```python
from build123d import *

# Parameters (mm, degrees)
SKETCH1_W                       = 63.5
SKETCH1_H                       = 44.45
BOSS_EXTRUDE1_DEPTH             = 6.35
LPATTERN1_COUNT                 = 2
LPATTERN1_PITCH                 = 55.88
TAP_DRILL_FOR_6_32_TAP1_D       = 2.7051
TAP_DRILL_FOR_6_32_TAP1_DEPTH   = 6.35
TAP_DRILL_FOR_6_32_TAP1_TIP     = 0.81269403
TAP_DRILL_FOR_6_32_TAP2_D       = 2.7051
TAP_DRILL_FOR_6_32_TAP2_DEPTH   = 6.35
TAP_DRILL_FOR_6_32_TAP2_TIP     = 0.81269403
TAP_DRILL_FOR_1_2_13_TAP1_D     = 10.71626
TAP_DRILL_FOR_1_2_13_TAP1_DEPTH = 6.35
TAP_DRILL_FOR_1_2_13_TAP1_TIP   = 3.219489309


with BuildPart() as part:
    # Sketch1 → Boss-Extrude1 (new body)
    with BuildSketch(Plane(origin=(0, 0, 0), x_dir=(1, 0, 0), z_dir=(0, 1, 0))):
        with Locations((4.75259427, -18.964156798)):
            Rectangle(SKETCH1_W, SKETCH1_H)
    extrude(amount=BOSS_EXTRUDE1_DEPTH)

    # Sketch16 → Tap Drill for #4-40 Tap1 (revolve, cut)
    with BuildSketch(Plane(origin=(-23.18740573, 0, 18.964156798), x_dir=(0, 0, -1), z_dir=(1, 0, 0))):
        Polygon((0, 0), (0, 13.379152758), (1.1303, 12.7), (1.1303, 0), align=None)
    tap_drill_for_4_40_tap1 = revolve(axis=Axis((-23.18740573, -6.35, 18.964156798), (0, 1, 0)), mode=Mode.SUBTRACT)

    # LPattern1: Tap Drill for #4-40 Tap1 ×2
    with Locations(*[(i * LPATTERN1_PITCH, 0, 0) for i in range(1, LPATTERN1_COUNT)]):
        add(tap_drill_for_4_40_tap1, mode=Mode.SUBTRACT)

    # Tap Drill for #6-32 Tap1
    with Locations(Plane.XY.offset(41.189156798)):
        with Locations((23.80259427, 3.175), (-14.29740573, 3.175)):
            Hole(TAP_DRILL_FOR_6_32_TAP1_D / 2, depth=TAP_DRILL_FOR_6_32_TAP1_DEPTH)
            with Locations((0, 0, -(TAP_DRILL_FOR_6_32_TAP1_DEPTH + TAP_DRILL_FOR_6_32_TAP1_TIP / 2))):  # 118° drill point
                Cone(0, TAP_DRILL_FOR_6_32_TAP1_D / 2, TAP_DRILL_FOR_6_32_TAP1_TIP, mode=Mode.SUBTRACT)

    # Tap Drill for #6-32 Tap2
    with Locations(Plane(origin=(0, 0, -3.260843202), x_dir=(-1, 0, 0), z_dir=(0, 0, -1))):
        with Locations((14.29740573, 3.175), (-23.80259427, 3.175)):
            Hole(TAP_DRILL_FOR_6_32_TAP2_D / 2, depth=TAP_DRILL_FOR_6_32_TAP2_DEPTH)
            with Locations((0, 0, -(TAP_DRILL_FOR_6_32_TAP2_DEPTH + TAP_DRILL_FOR_6_32_TAP2_TIP / 2))):  # 118° drill point
                Cone(0, TAP_DRILL_FOR_6_32_TAP2_D / 2, TAP_DRILL_FOR_6_32_TAP2_TIP, mode=Mode.SUBTRACT)

    # Tap Drill for 1/2-13 Tap1
    with Locations(Plane(origin=(0, 6.35, 0), x_dir=(-1, 0, 0), z_dir=(0, 1, 0))):
        with Locations((-4.75259427, 18.964156798)):
            Hole(TAP_DRILL_FOR_1_2_13_TAP1_D / 2, depth=TAP_DRILL_FOR_1_2_13_TAP1_DEPTH)
            with Locations((0, 0, -(TAP_DRILL_FOR_1_2_13_TAP1_DEPTH + TAP_DRILL_FOR_1_2_13_TAP1_TIP / 2))):  # 118° drill point
                Cone(0, TAP_DRILL_FOR_1_2_13_TAP1_D / 2, TAP_DRILL_FOR_1_2_13_TAP1_TIP, mode=Mode.SUBTRACT)


solid = part.part
```
The listing builds one solid part. Answer for the finished solid, in the listing's coordinates (mm). A direction names the side the tool comes from. Round coordinates to 2 decimals unless told otherwise and drop trailing zeros. Loops run counter-clockwise (first coordinate to the right, second up) from the corner with the lowest first, then second, coordinate; pieces in that order, holes last.
1) A cutting plane is placed at B-B on x = 6. Determine the outline of the cut face in (y, z).
Outcome:
outline: (0, -3.26) - (6.35, -3.26) - (6.35, 13.75) - (0, 13.75) - close; (0, 24.18) - (6.35, 24.18) - (6.35, 41.19) - (0, 41.19) - close
2) A cutting plane is placed at C-C on z = 2. Determine the outline of the cut face in (x, y) (3 decimals), plus the area to 3 significant figures.
Outcome:
outline: (-26.997, 0) - (36.503, 0) - (36.503, 6.35) - (-26.997, 6.35) - close; hole circle Ø2.705 at (-14.297, 3.175); hole circle Ø2.705 at (23.803, 3.175)
area: 392 mm2
3) For faces 1 (the face through (-26.997, 3, 19)), 2 (the face through (-13.007, 3.581, -0.041)), 3 (the face through (-12.946, 3.234, 37.97)), determine the directions among +Z, -Z, +X, -X, +Y, -Y from which every point of the face is accessible in a straight line to the end or side of a thin tool.
Outcome:
face 1: +Z, -Z, -X, +Y, -Y
face 2: -Z
face 3: +Z
4) For a pull along Y with two mould halves and no side action, classify faces 4 (the face through (31.74, 3.131, 18.357)), 5 (the face through (11, 0, 19)), 6 (the face through (25.154, 3.234, 37.97)) as released by +Y, released by -Y, zero draft, split by the parting line, or undercut.
Outcome:
face 4: zero draft
face 5: released by -Y
face 6: undercut
5) A cutting plane is placed at A-A on y = 1. Determine the outline of the cut face in (x, z).
Outcome:
outline: (-27, -3.26) - (36.5, -3.26) - (36.5, 41.19) - (-27, 41.19) - close; hole circle Ø2.26 at (-23.19, 18.96); hole circle Ø10.72 at (4.75, 18.96); hole circle Ø2.26 at (32.69, 18.96)
6) Given P1, Ø2, axis at x = -14.3, y = 3.18, coming from the -Z side; P2, Ø2, axis at x = 32.69, z = 18.96, coming from the +Y side; P3, Ø2, axis at x = 23.8, y = 3.18, coming from the +Z side, each flat-ended and moving along its own axis, determine where each tip first touches the part or whether it passes through.
Outcome:
P1: stops at z = 3.3
P2: passes through
P3: stops at z = 34.63
7) Consider line 1 (Z direction, x = 3.5, y = 5); line 2 (Z direction, x = -24, y = 5.25). Determine where each line is inside the solid, lowest interval first.
Outcome:
line 1: z = -3.26 to 13.75, 24.17 to 41.19
line 2: z = -3.26 to 18.18, 19.75 to 41.19
